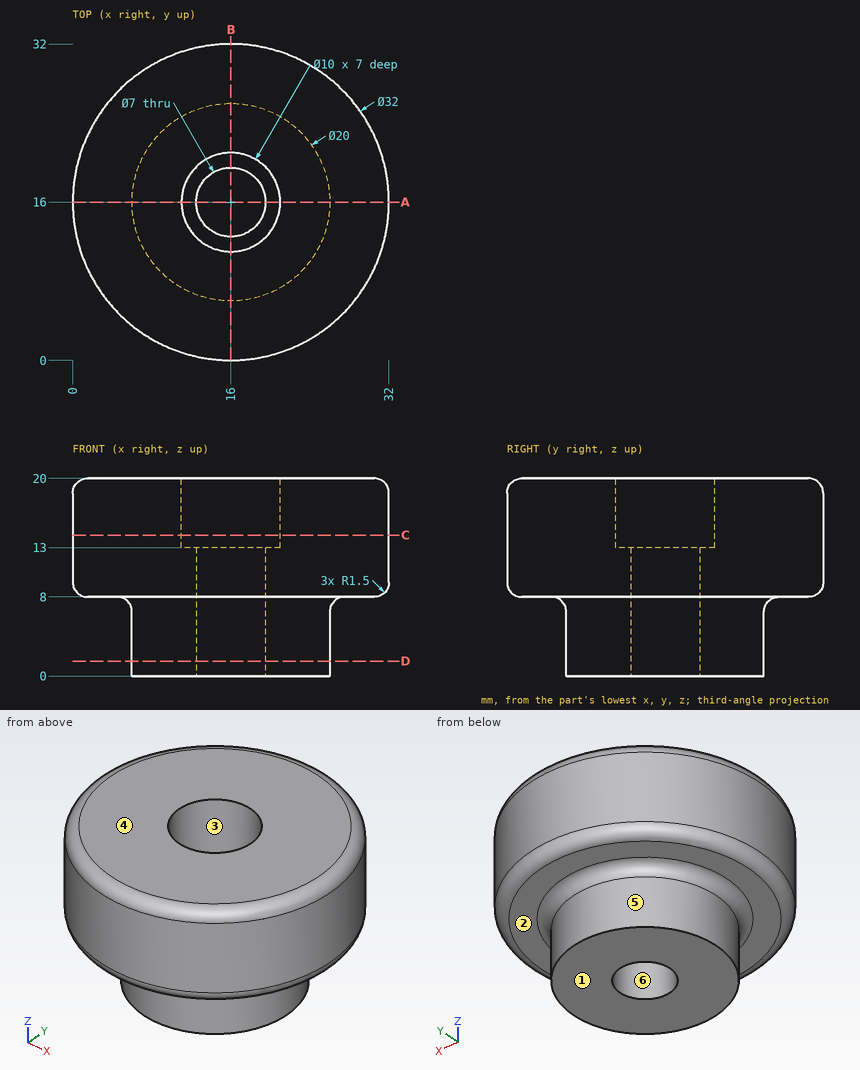
Geometry check sheet. Reference: drawing and pictorial views, mm from the part's lowest x, y, z. A direction names the side the tool comes from. Give positions to 0.01 mm unless a question says otherwise; leave off trailing zeros. Order: outer loops, then holes, each group sorted by start corner. A loop starts at its lowest first (then second) coordinate and runs counter-clockwise, first axis right, second up. Notation, with made-up numbers: M 34,59 L 90,59 A10 cw 90,75 Z; hole C 4,-13 d3. An arc over 180 degrees is marked long. Return JSON: item names as keys, results as strings. Group by question number.
1) Mould release check, pull along Y, two halves, no side actions. Record for the marked faces 4, 5 and 6: pulls with the +Y half, pulls with the -Y half, needs draft (parallel to the pull), parting line crosses it, or undercut.
2) Scan lines: line 1 (Y direction, x = 16, z = 17.75); line 2 (Z direction, x = 30, y = 13); line 3 (Y direction, x = 16, z = 9.5). Record each from-to range of solid material in increasing order.
3) Go/stop test with flat-tipped pins: pin 1 Ø3 at (y, z) = (22, 3) entering from +X; pin 2 Ø6 at (y, z) = (8, 4) entering from +X; pin 3 Ø1.5 at (y, z) = (11.5, 16) entering from +X. Record where each tip stops, or that it passes through.
4) Access from +Z, -Z, +X, -X, +Y, -Y to the whole of each face (thin tool, end or side, straight path). Record for the marked faces 1, 2 and 3.
5) Section check A-A on y = 16. Record the cut outline in (x, z).
6) Section check D-D on z = 1.5. Record the cut outline in (x, y), and give its area (3 significant figures).
7) Section check C-C on z = 14.25. Record the cut outline in (x, y), and give its area (3 significant figures).
Answer block:
{
 "1": {"face 4": "needs draft", "face 5": "parting line crosses it", "face 6": "undercut"},
 "2": {"line 1": "y = 0 to 11, 21 to 32", "line 2": "z = 8 to 20", "line 3": "y = 0 to 12.5, 19.5 to 32"},
 "3": {"pin 1": "stops at x = 24.93", "pin 2": "stops at x = 24.66", "pin 3": "stops at x = 31.55"},
 "4": {"face 1": "-Z, +X, -X, +Y, -Y", "face 2": "-Z", "face 3": "+Z"},
 "5": {"outline": "M 0,9.5 A1.5 ccw 1.5,8 L 4.5,8 A1.5 cw 6,6.5 L 6,0 L 12.5,0 L 12.5,13 L 11,13 L 11,20 L 1.5,20 A1.5 ccw 0,18.5 Z; M 19.5,0 L 26,0 L 26,6.5 A1.5 cw 27.5,8 L 30.5,8 A1.5 ccw 32,9.5 L 32,18.5 A1.5 ccw 30.5,20 L 21,20 L 21,13 L 19.5,13 Z"},
 "6": {"outline": "C 16,16 d20; hole C 16,16 d7", "area": "276 mm^2"},
 "7": {"outline": "C 16,16 d32; hole C 16,16 d10", "area": "726 mm^2"}
}
